Could you check a few things on this model? Use its own coordinates, in mm. Face numbers are marked on the shaded views. A direction names the side the tool comes from. Round coordinates to 2 decimals unless told otherwise and drop trailing zeros. Order: outer loops, then holes, each group sorted by start corner. A loop starts at its lowest first (then second) coordinate and runs counter-clockwise, first axis right, second up. Notation, with made-up numbers: (-35.75, 6) - (-11.75, 6) arc R35 cw to (-11.75, 43) - close; hole circle Ø10 at (79.25, 73). An arc over 180 degrees is marked (long way). Return JSON: item names as keys, results as strings. Group by question number.
from build123d import *

# Parameters (mm, degrees)
BOSS_EXTRUDE1_DEPTH = 12.5
BOSS_EXTRUDE2_DEPTH = 4.02005
FILLET2_R           = 2


with BuildPart() as part:
    # Sketch2 → Boss-Extrude1 (new, symmetric)
    with BuildSketch(Plane.XY):
        Polygon((29.367996497, -11.749519802), (29.367996497, -35.249519802), (33.388046748, -35.249519802), (33.388046748, -47.391114069), (8.625661213, -49.557542086), (8.625661213, -54.557542086), (33.388046748, -56.723970102), (43.388046748, -56.723970102), (43.388046748, -11.749519802), align=None)
    extrude(amount=BOSS_EXTRUDE1_DEPTH, both=True)

    # Sketch4 → Boss-Extrude2 (add)
    with BuildSketch(Plane.ZY.offset(-33.388046748)):
        with BuildLine():
            Line((-12.5, -35.249519802), (-12.5, -47.391114069))
            Line((-12.5, -47.391114069), (-12.494860757, -47.391114069))
            ThreePointArc((-12.494860757, -47.391114069), (-8.711197631, -38.784864994), (0, -35.249519802))
            Line((0, -35.249519802), (-12.5, -35.249519802))
        make_face()
        with BuildLine():
            Line((12.5, -35.249519802), (0, -35.249519802))
            ThreePointArc((0, -35.249519802), (8.711197631, -38.784864994), (12.494860757, -47.391114069))
            Line((12.494860757, -47.391114069), (12.5, -47.391114069))
            Line((12.5, -47.391114069), (12.5, -35.249519802))
        make_face()
    extrude(amount=BOSS_EXTRUDE2_DEPTH)

    # Sketch3 → Cut-Revolve1 (revolve, cut)
    with BuildSketch(Plane.ZY.offset(-25.388046748)):
        with BuildLine():
            Line((-12.5, -30.749519802), (12.5, -30.749519802))
            Line((12.5, -30.749519802), (12.5, -12.949519802))
            ThreePointArc((12.5, -12.949519802), (0, -25.449519802), (-12.5, -12.949519802))
            Line((-12.5, -12.949519802), (-12.5, -30.749519802))
        make_face()
    revolve(axis=Axis((25.388046748, -30.749519802, -12.5), (0, 0, 1)), mode=Mode.SUBTRACT)

    # Fillet2
    fillet2_edges = [part.edges().sort_by_distance(p)[0] for p in [
        (29.367996497, -11.749519802, 0),
        (8.625661213, -49.557542086, 0),
        (8.625661213, -54.557542086, 0),
    ]]
    fillet(fillet2_edges, radius=FILLET2_R)


solid = part.part
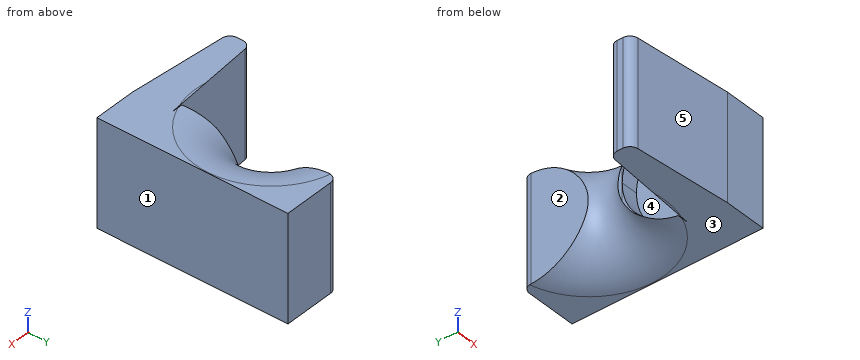
1) I want a section at A-A, the plane z = -10.5. List the corners of the cut face in (x, y) for me.
2) We'd pull the mould along Z, two halves only. Please class the marked faces 3, 4 and 5: +Z half, -Z half, draft (parallel to the pull), parting line (faces both ways), or undercut.
3) I want a section at C-C, the plane z = 2.25. List the corners of the cut face in (x, y) for me.
4) For the marked faces 1 and 2, which set-ups out of +Z, -Z, +X, -X, +Y, -Y let a thin tool reach every point of the face, with its end or its side?
5) I want a section at D-D, the plane x = 18. List the corners of the cut face in (y, z) for me.
6) I want a section at B-B, the plane x = 14. List the corners of the cut face in (y, z) for me.
7) If I drill on line 1 along Y through (x, z) = (31, 6); line 2 along X through (y, z) = (-14, 4.75); line 3 along X through (y, z) = (-47, 10), over which ranges is the centre line in solid material (lowest first)? Write a range as from..to.
8) Will these pins go through, and if not, where does the flat tip stop? pin 1 (8 mm diameter, centred on x = 28.5, z = 5.5, fed in from -Y); pin 2 (6 mm diameter, centred on y = -18, z = -3.5, fed in from -X); pin 3 (1.5 mm diameter, centred on y = -38, z = 3.5, fed in from -X); pin 4 (8 mm diameter, centred on x = 24.5, y = -36.5, fed in from +Z).
Outcome:
{
 "1": {"outline": "(8.63, -52.72) arc R2 ccw to (10.45, -54.72) - (33.39, -56.72) - (43.39, -56.72) - (43.39, -11.75) - (31.37, -11.75) arc R2 ccw to (29.37, -13.75) - (29.37, -20.48) arc R11.02 cw to (29.51, -40.97) - (33.39, -40.97) - (33.39, -47.39) - (10.45, -49.4) arc R2 ccw to (8.63, -51.39) - close"},
 "2": {"face 3": "-Z half", "face 4": "undercut", "face 5": "draft"},
 "3": {"outline": "(8.63, -52.72) arc R2 ccw to (10.45, -54.72) - (33.39, -56.72) - (43.39, -56.72) - (43.39, -11.75) - (31.37, -11.75) arc R2 ccw to (29.37, -13.75) - (29.37, -26.95) arc R5.5 cw to (29.37, -34.55) - (29.37, -35.45) - (33.39, -35.45) - (33.39, -47.39) - (10.45, -49.4) arc R2 ccw to (8.63, -51.39) - close"},
 "4": {"face 1": "+Z, -Z, +X, +Y, -Y", "face 2": "+Z, -Z, -X, +Y"},
 "5": {"outline": "(-55.38, -12.5) - (-48.74, -12.5) - (-48.74, 12.5) - (-55.38, 12.5) - close"},
 "6": {"outline": "(-55.03, -12.5) - (-49.09, -12.5) - (-49.09, 12.5) - (-55.03, 12.5) - close"},
 "7": {"line 1": "-56.52..-47.6, -36.78..-34.65, -26.85..-11.78", "line 2": "29.37..43.39", "line 3": "33.39..43.39"},
 "8": {"pin 1": "y = -56.65", "pin 2": "x = 29.37", "pin 3": "x = 33.39", "pin 4": "through"}
}
